```python
from build123d import *

# Parameters (mm, degrees)
F0_W        = 20
F0_H        = 32
F1_DEPTH    = 3
F2_W        = 2.5
F2_H        = 32
F3_DEPTH    = 9
F4_R        = 2.8970562748
F5_W        = 4
F5_H        = 16
F6_DEPTH    = 5
F7_R        = 1
F8_DEPTH    = 25
F9_T1_DEPTH = 26.8639610307


# Not quite as in the source:
# - a fillet or chamfer that OpenCascade refuses, or shapes differently, is made with other operations: its cross-section is extruded or revolved along the edge and cut away or added


with BuildPart() as f1:
    # F0 (on Top) → F1 (new body)
    with BuildSketch(Plane.XY):
        with Locations((-10, 0)):
            Rectangle(F0_W, F0_H)
    extrude(amount=F1_DEPTH)

    # F2 (on face) → F3 (join)
    with BuildSketch(Plane(origin=(0, 0, 0), x_dir=(1, 0, 0), z_dir=(0, 0, -1))):
        with Locations((-18.75, 0)):
            Rectangle(F2_W, F2_H)
    extrude(amount=F3_DEPTH)

    # F4
    f4_edges = [f1.edges().sort_by_distance(p)[0] for p in [
        (0, 0, 0),
    ]]
    fillet(f4_edges, radius=F4_R)

    # F5 (on face) → F6 (join)
    with BuildSketch(Plane.XY.offset(3)):
        with Locations((-2, 8)):
            Rectangle(F5_W, F5_H)
    extrude(amount=F6_DEPTH)

    # F7 (on face) → F8 (cut)
    with BuildSketch(Plane.XZ):
        with Locations((-1.9916295272, 5.9999883225)):
            Circle(F7_R)
    extrude(amount=-F8_DEPTH, mode=Mode.SUBTRACT)

    # F9: fillet of radius 2.1727922061 on 2 edges, made by hand

    # F9_s2 → F9_t1 (cut)
    with BuildSketch(Plane.XZ.offset(-21.4319805153)):
        with BuildLine():
            ThreePointArc((-1.8272077939, 8), (-3.3636038969, 7.3636038969), (-4, 5.8272077939))
            Line((-4, 5.8272077939), (-4, 8))
            Line((-4, 8), (-1.8272077939, 8))
        make_face()
        with BuildLine():
            ThreePointArc((0, 5.8272077939), (-0.6363961031, 7.3636038969), (-2.1727922061, 8))
            Line((-2.1727922061, 8), (0, 8))
            Line((0, 8), (0, 5.8272077939))
        make_face()
    extrude(amount=F9_T1_DEPTH, mode=Mode.SUBTRACT)


solid = f1.part
```
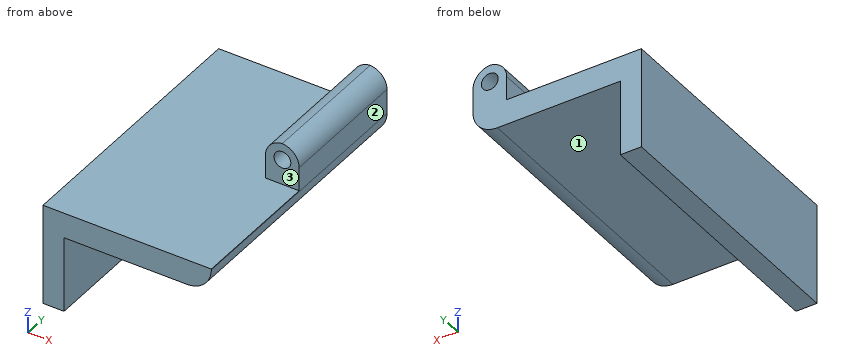
For this review, take the finished solid that the model builds, in its own axes (mm). Face numbers are marked on the shaded views. A direction names the side the tool comes from. Coordinates: 2 decimals unless noted, no trailing zeros. Write each loop counter-clockwise with the first axis right and the second up, starting at its lowest first coordinate (ties: lowest second). Pieces come first, ordered by that corner, then holes. Notation, with made-up numbers: (-37, 9.5) - (-24, 9.5) arc R31 ccw to (-24, 36.5) - close; hole circle Ø4 at (33.25, 73.25). An arc over 180 degrees is marked (long way). Answer in a Markdown table with one row per item. Add a question column.
Q1. For P1, Ø12, axis at x = -7.5, y = -10.5, coming from the +Z side; P2, Ø12, axis at x = -8, y = -8, coming from the -Z side; P3, Ø1.4, axis at y = 5.5, z = 4, coming from the -X side, all flat-tipped, find the tip position at first contact; note any pin that passes through.
Q2. We need section A-A, the plane y = -4.5. State the section outline as (x, z) points, and give its area (3 significant figures).
Q3. We need section D-D, the plane y = 5. State the section outline as (x, z) points.
Q4. Tool access review of the marked faces 1, 2 and 3: name each direction out of +Z, -Z, +X, -X, +Y, -Y from which nothing blocks a thin tool from reaching the whole face with its end or side.
Q5. We need section B-B, the plane z = 6.5. State the section outline as (x, y) points.
Q6. We need section C-C, the plane x = -5.5. State the section outline as (y, z) points, and give its area (3 significant figures).
Q7. For probe 1 along X at (y, z) = (11, -4.5); probe 2 along Z at (x, y) = (-14.75, -7); probe 3 along Z at (x, y) = (-18, -1), list the stretches that pass through material, from the lowest coordinate up.
Answer list:
| question | item | result |
|---|---|---|
| 1 | P1 | stops at z = 3 |
| 1 | P2 | stops at z = 0 |
| 1 | P3 | stops at x = -4 |
| 2 | outline | (-20, -9) - (-17.5, -9) - (-17.5, 0) - (-2.9, 0) arc R2.9 ccw to (0, 2.9) - (0, 3) - (-20, 3) - close |
| 2 | area | 80.7 mm2 |
| 3 | outline | (-20, -9) - (-17.5, -9) - (-17.5, 0) - (-2.9, 0) arc R2.9 ccw to (0, 2.9) - (0, 5.83) arc R2.17 ccw to (-2, 7.99) arc R2.17 ccw to (-4, 5.83) - (-4, 3) - (-20, 3) - close; hole circle Ø2 at (-1.99, 6) |
| 4 | face 1 | -Z, +X, +Y, -Y |
| 4 | face 2 | +Z, -Z, +X, +Y, -Y |
| 4 | face 3 | +Z, +X, -X, -Y |
| 5 | outline | (-3.89, 0) - (-2.86, 0) - (-2.86, 16) - (-3.89, 16) - close; (-1.13, 0) - (-0.11, 0) - (-0.11, 16) - (-1.13, 16) - close |
| 6 | outline | (-16, 0) - (16, 0) - (16, 3) - (-16, 3) - close |
| 6 | area | 96.0 mm2 |
| 7 | probe 1 | x = -20 to -17.5 |
| 7 | probe 2 | z = 0 to 3 |
| 7 | probe 3 | z = -9 to 3 |
